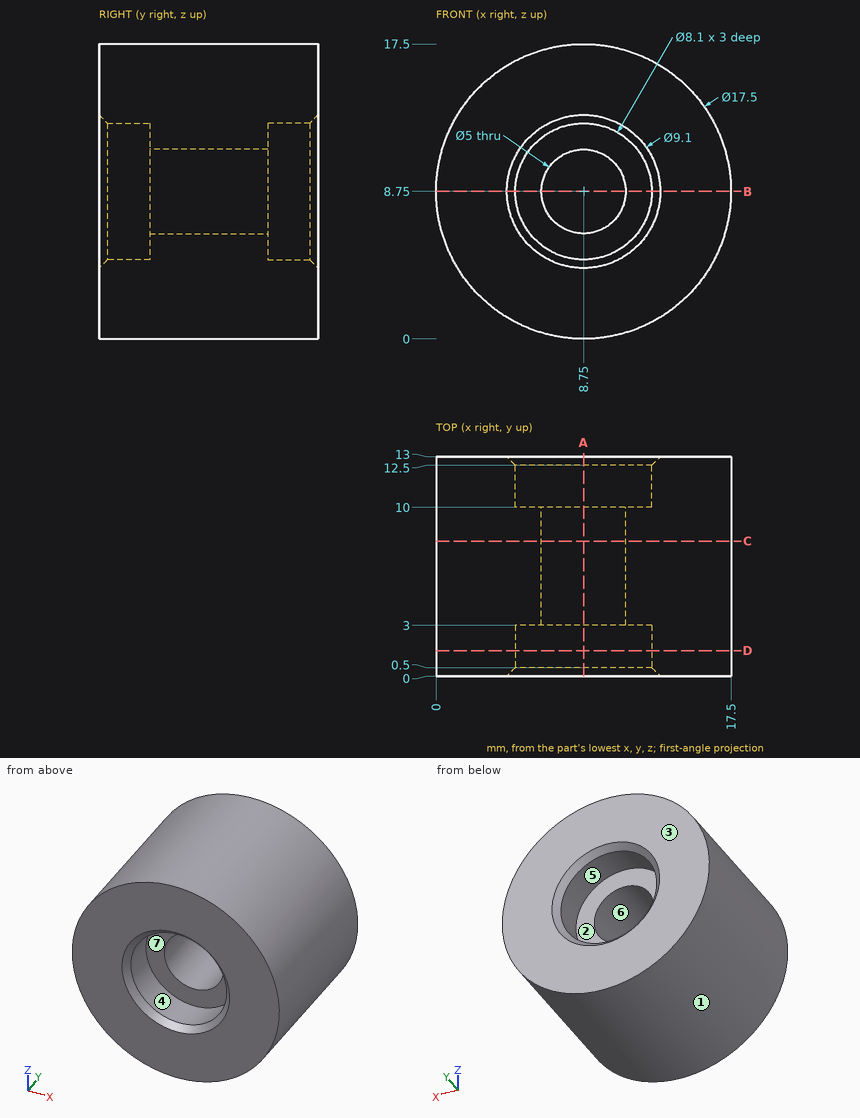
The drawing under review shows one solid part. Ordinate dimensions are in mm from its lowest x, y, z. A direction names the side the tool comes from. Round coordinates to 2 decimals unless told otherwise and drop trailing zeros. Loops run counter-clockwise (first coordinate to the right, second up) from the corner with the lowest first, then second, coordinate; pieces in that order, holes last. Notation, with made-up numbers: (32.5, -25.5) -> (73.5, -25.5) arc R16 cw to (73.5, -8.5) -> close; hole circle Ø11 at (-25, 0). An arc over 180 degrees is marked (long way). Answer in a Markdown table with one row per item.
1) Consider section A-A, the plane x = 8.75. Write out the cut boundary in (y, z), plus the area to 3 significant figures.
Taken from the geometry:
| item | result |
|---|---|
| outline | (0, 0) -> (13, 0) -> (13, 4.2) -> (12.5, 4.7) -> (10, 4.7) -> (10, 6.25) -> (3, 6.25) -> (3, 4.7) -> (0.5, 4.7) -> (0, 4.2) -> close; (0, 13.3) -> (0.5, 12.8) -> (3, 12.8) -> (3, 11.25) -> (10, 11.25) -> (10, 12.8) -> (12.5, 12.8) -> (13, 13.3) -> (13, 17.5) -> (0, 17.5) -> close |
| area | 143 mm² |
2) For pin 1 Ø2.5 at (x, z) = (8.5, 10.5) entering from +Y; pin 2 Ø1 at (x, z) = (7, 10) entering from -Y; pin 3 Ø1.5 at (y, z) = (8.5, 3.5) entering from +X, all flat-tipped, find the tip position at first contact; note any pin that passes through.
Taken from the geometry:
| item | result |
|---|---|
| pin 1 | stops at y = 10 |
| pin 2 | stops at y = 3 |
| pin 3 | stops at x = 16.25 |
3) Wall thickness on line 1 along X through (y, z) = (2, 8.75); line 2 along X through (y, z) = (5, 8.75); line 3 along Z through (x, y) = (8.25, 4): over which ranges is each line inside the solid? List them lowest first.
Taken from the geometry:
| item | result |
|---|---|
| line 1 | x = 0 to 4.7, 12.8 to 17.5 |
| line 2 | x = 0 to 6.25, 11.25 to 17.5 |
| line 3 | z = 0.01 to 6.3, 11.2 to 17.49 |
4) Consider section D-D, the plane y = 1.5. Write out the cut boundary in (x, z), plus the area to 3 significant figures.
Taken from the geometry:
| item | result |
|---|---|
| outline | circle Ø17.5 at (8.75, 8.75); hole circle Ø8.1 at (8.75, 8.75) |
| area | 189 mm² |
5) Tool access review of the marked faces 5, 6 and 7: name each direction out of +Z, -Z, +X, -X, +Y, -Y from which nothing blocks a thin tool from reaching the whole face with its end or side.
Taken from the geometry:
| item | result |
|---|---|
| face 5 | +Y |
| face 6 | +Y, -Y |
| face 7 | -Y |
6) Draft analysis for pull direction Z (two halves, no side actions). For the marked faces 1, 2, 3 and 4, state which applies: pulls with the +Z half, pulls with the -Z half, needs draft (parallel to the pull), parting line crosses it, or undercut.
Taken from the geometry:
| item | result |
|---|---|
| face 1 | parting line crosses it |
| face 2 | undercut |
| face 3 | needs draft |
| face 4 | undercut |
7) Consider section C-C, the plane y = 8. Write out the cut boundary in (x, z).
Taken from the geometry:
| item | result |
|---|---|
| outline | circle Ø17.5 at (8.75, 8.75); hole circle Ø5 at (8.75, 8.75) |
8) Consider section B-B, the plane z = 8.75. Write out the cut boundary in (x, y), plus the area to 3 significant figures.
Taken from the geometry:
| item | result |
|---|---|
| outline | (0, 0) -> (4.2, 0) -> (4.7, 0.5) -> (4.7, 3) -> (6.25, 3) -> (6.25, 10) -> (4.7, 10) -> (4.7, 12.5) -> (4.2, 13) -> (0, 13) -> close; (11.25, 3) -> (12.8, 3) -> (12.8, 0.5) -> (13.3, 0) -> (17.5, 0) -> (17.5, 13) -> (13.3, 13) -> (12.8, 12.5) -> (12.8, 10) -> (11.25, 10) -> close |
| area | 143 mm² |
